The figure shows three views and two pictorial views of one solid part (mm, origin at its lowest corner). Answer the questions. Round coordinates to 2 decimals unless told otherwise and drop trailing zeros. Write each loop counter-clockwise with the first axis right and the second up, starting at its lowest first coordinate (ties: lowest second). Pieces come first, ordered by that corner, then holes.
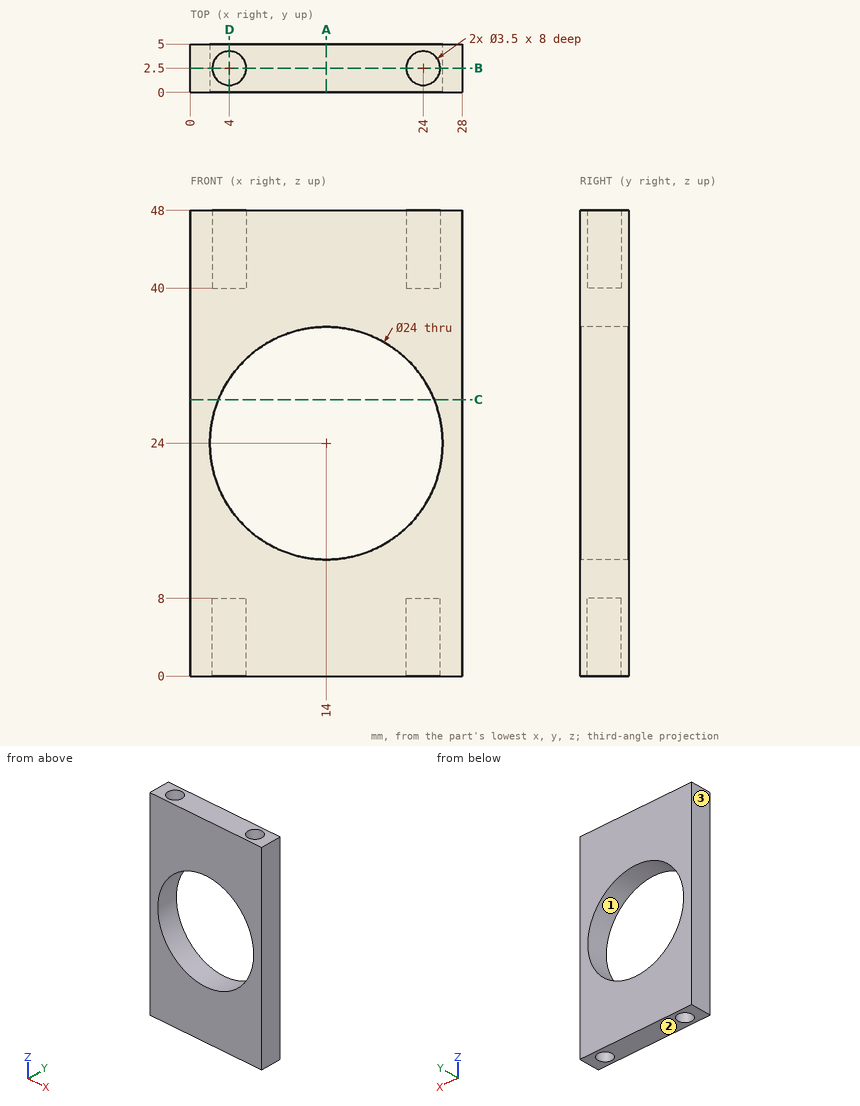
Q1. Section B-B (y = 2.5) is taken. Determine the outline of the cut face in (x, z), then the cut area to 3 significant figures.
Verdict:
outline: (0, 0) - (2.25, 0) - (2.25, 8) - (5.75, 8) - (5.75, 0) - (22.25, 0) - (22.25, 8) - (25.75, 8) - (25.75, 0) - (28, 0) - (28, 48) - (25.75, 48) - (25.75, 40) - (22.25, 40) - (22.25, 48) - (5.75, 48) - (5.75, 40) - (2.25, 40) - (2.25, 48) - (0, 48) - close; hole circle Ø24 at (14, 24)
area: 780 mm2
Q2. Section D-D (x = 4) is taken. Determine the outline of the cut face in (y, z), then the cut area to 3 significant figures.
Verdict:
outline: (0, 0) - (0.75, 0) - (0.75, 8) - (4.25, 8) - (4.25, 0) - (5, 0) - (5, 17.37) - (0, 17.37) - close; (0, 30.63) - (5, 30.63) - (5, 48) - (4.25, 48) - (4.25, 40) - (0.75, 40) - (0.75, 48) - (0, 48) - close
area: 118 mm2
Q3. Section A-A (x = 14) is taken. Determine the outline of the cut face in (y, z), then the cut area to 3 significant figures.
Verdict:
outline: (0, 0) - (5, 0) - (5, 12) - (0, 12) - close; (0, 36) - (5, 36) - (5, 48) - (0, 48) - close
area: 120 mm2
Q4. Straight lines are drawn through the part: probe 1 along X at (y, z) = (2.5, 46); probe 2 along Y at (x, z) = (24, 4.75); probe 3 along Z at (x, y) = (3, 2.9). For each, find the intervals that lie inside material, in ascending order.
Verdict:
probe 1: x = 0 to 2.25, 5.75 to 22.25, 25.75 to 28
probe 2: y = 0 to 0.75, 4.25 to 5
probe 3: z = 8 to 19.2, 28.8 to 40
Q5. Determine the mould class of the marked faces 1, 2 and 3 for opening direction X: pulls with the +X half, pulls with the -X half, needs draft (parallel to the pull), parting line crosses it, or undercut.
Verdict:
face 1: undercut
face 2: needs draft
face 3: pulls with the -X half
Q6. Section C-C (z = 28.5) is taken. Determine the outline of the cut face in (x, y).
Verdict:
outline: (0, 0) - (2.88, 0) - (2.88, 5) - (0, 5) - close; (25.12, 0) - (28, 0) - (28, 5) - (25.12, 5) - close
Q7. Flat-ended cylindrical pins translate along their axes: pin 1 Ø1.8 at (x, y) = (4, 3) entering from -Z; pin 2 Ø1 at (x, y) = (23.5, 1.5) entering from +Z; pin 3 Ø14.5 at (x, z) = (14, 24) entering from +Y. Find the tip coordinate at first contact, or state that the pin passes through.
Verdict:
pin 1: stops at z = 8
pin 2: stops at z = 40
pin 3: passes through
